Input: part model. Units: mm. Frame: model coordinates. A direction names the side the tool comes from. Give positions to 0.01 mm unless a question says otherwise; leave off trailing zeros. Loops run counter-clockwise (first coordinate to the right, second up) from the corner with the lowest first, then second, coordinate; pieces in that order, holes last. Notation, with made-up numbers: (-34.75, -16.5) -> (-22.75, -16.5) arc R19 cw to (-22.75, -0.5) -> close; hole circle Ø8 at (-31.5, 40). An arc over 180 degrees is marked (long way). Use CSV: the item, a comma, the result in double quotes.
```python
from build123d import *

# Parameters (mm, degrees)
SKETCH2_R           = 4
SKETCH1_R           = 4.5
SKETCH1_35_R        = 4.5
SKETCH1_35_R_2      = 3.5
BOSS_EXTRUDE1_DEPTH = 2
CUT_EXTRUDE1_DEPTH  = 10


with BuildPart() as part:
    # Sketch2 → Loft1 section 0
    with BuildSketch(Plane(origin=(0, 13, 0), x_dir=(1, 0, 0), z_dir=(0, 1, 0))):
        Circle(SKETCH2_R)
    # Sketch1 → Loft1 section 1
    with BuildSketch(Plane(origin=(0, 0, 0), x_dir=(1, 0, 0), z_dir=(0, 1, 0))):
        Circle(SKETCH1_R)
    loft()

    # Sketch1_35 → Boss-Extrude1 (add)
    # profile 1 of 2: a face of its own
    with BuildSketch(Plane(origin=(0, 0, 0), x_dir=(1, 0, 0), z_dir=(0, 1, 0))):
        with BuildLine():
            Line((0, 7.392655237), (-1.626288958, 4.195853218))
            ThreePointArc((-1.626288958, 4.195853218), (0, 4.5), (1.626288958, 4.195853218))
            Line((1.626288958, 4.195853218), (0, 7.392655237))
        make_face()
    # profile 2 of 2: a face of its own
    with BuildSketch(Plane(origin=(0, 0, 0), x_dir=(1, 0, 0), z_dir=(0, 1, 0))):
        Circle(SKETCH1_35_R)
        Circle(SKETCH1_35_R_2, mode=Mode.SUBTRACT)
    extrude(amount=BOSS_EXTRUDE1_DEPTH)

    # Sketch1_36 → Cut-Extrude1 (cut)
    with BuildSketch(Plane(origin=(0, 0, 0), x_dir=(1, 0, 0), z_dir=(0, 1, 0))):
        with BuildLine():
            Line((3.47706773, -0.4), (-3.47706773, -0.4))
            ThreePointArc((-3.47706773, -0.4), (0, -3.5), (3.47706773, -0.4))
        make_face()
        with BuildLine():
            ThreePointArc((3.47706773, 0.4), (0, 3.5), (-3.47706773, 0.4))
            Line((-3.47706773, 0.4), (3.47706773, 0.4))
        make_face()
    extrude(amount=CUT_EXTRUDE1_DEPTH, mode=Mode.SUBTRACT)


solid = part.part
```
1) Reachability of faces 1 (the flat face through (0, 0, 0)), 2 (the flat face through (0, 2, -5)), 3 (the flat face through (0, 10, 2)) from +Z, -Z, +X, -X, +Y, -Y: full face, straight path, thin tool, end or side. Return the list, or none.
From the geometry:
face 1,"+Z, -Z, +X, -X, -Y"
face 2,"+Y"
face 3,"-Y"
2) Contact query for flat-ended pins moving along their axis: pin 1 (2 mm diameter, centred on x = -1.5, y = 5.5, fed in from -Z); pin 2 (3 mm diameter, centred on y = 4, z = -1, fed in from -X); pin 3 (1.6 mm diameter, centred on x = 1.5, z = -2, fed in from -Y). Output: stop coordinate, or through.
From the geometry:
pin 1,"stops at z = -4.27"
pin 2,"stops at x = -4.39"
pin 3,"stops at y = 10"
3) Mould query, pull axis X, two halves, no side actions, for faces 4 (the conical face through (4.02, 7.42, -1.27)), 5 (the flat face through (0, 13, 0)), 6 (the flat face through (0, 5, -0.4)), 7 (the cylindrical face through (-0.1, 4.9, 3.5)). Classes: pulls with the +X half, pulls with the -X half, needs draft (parallel to the pull), parting line crosses it, or undercut.
From the geometry:
face 4,"parting line crosses it"
face 5,"needs draft"
face 6,"undercut"
face 7,"undercut"
4) Ray query, line 1 (Z direction, x = -1, y = 6.5); line 2 (Z direction, x = -2.75, y = 2.5); line 3 (X direction, y = 6.25, z = 1.5). Return the intervals inside material, ascending.
From the geometry:
line 1,"z = -4.13 to -3.35, -0.4 to 0.4, 3.35 to 4.13"
line 2,"z = -3.44 to -2.17, -0.4 to 0.4, 2.17 to 3.44"
line 3,"x = -3.99 to -3.16, 3.16 to 3.99"
5) Section query A-A (y = 4.5). Return loops of the section in (x, z).
From the geometry:
outline,"circle Ø8.65 at (0, 0); hole (-3.48, -0.4) arc R3.5 ccw to (3.48, -0.4) -> close; hole (-3.48, 0.4) -> (3.48, 0.4) arc R3.5 ccw to start"
